Verification items for the finished model (mm, model axes). A direction names the side the tool comes from. Round coordinates to 2 decimals unless told otherwise and drop trailing zeros. Write each loop counter-clockwise with the first axis right and the second up, starting at its lowest first coordinate (ties: lowest second). Pieces come first, ordered by that corner, then holes. Notation, with made-up numbers: (-18, -32) -> (9, -32) arc R30 ccw to (9, -4) -> close; hole circle Ø9 at (9.5, 20). An arc over 180 degrees is marked (long way). Answer as a JSON object with one key per item and string values. Group by question number.
(1) Sectioned sample at B-B on y = 21.5. Record the cut outline in (x, z).
(2) Sectioned sample at A-A on z = 14. Record the cut outline in (x, y).
(3) Draft check along X on faces 5 (the face through (35, 15, 14)), 6 (the face through (6, 30, 14)), 7 (the face through (6.11, 16.01, 4.93)). Enter one of: released by +X, released by -X, zero draft, split by the parting line, or undercut.
(4) Scan lines: L1, parallel to Y at x = 5.5, z = 23.25; L2, parallel to Z at x = 17.5, y = 23; L3, parallel to X at y = 18.75, z = 14. Record each from-to range of solid material in increasing order. Write a range as from..to.
(5) Sectioned sample at C-C on x = 22. Record the cut outline in (y, z).
(6) Gauge pin test, flat ends, axial feed: pin 1 Ø3 at (x, y) = (5.5, 24) entering from +Z; pin 2 Ø6.5 at (x, z) = (16, 10.5) entering from +Y; pin 3 Ø1.5 at (x, z) = (25, 13.5) entering from +Y. Record the tip position at first contact, or that the pin passes through.
(7) Sectioned sample at D-D on y = 12. Record the cut outline in (x, z).
(8) Set-up check for faces 1 (the face through (31.408, 6.601, 24.549)), 2 (the face through (23, 8, 17)), 3 (the face through (16, 21, 6)), 4 (the face through (5, 15, 10)): record each of +Z, -Z, +X, -X, +Y, -Y from which the full face is reachable in a straight line by a thin tool's end or side.
```python
from build123d import *

# Parameters (mm, degrees)
SKETCH1_W           = 35
SKETCH1_H           = 30
BOSS_EXTRUDE1_DEPTH = 28
SKETCH2_R           = 2
CUT_EXTRUDE1_DEPTH  = 7
SKETCH4_R           = 7
CUT_EXTRUDE2_DEPTH  = 8
SKETCH5_R           = 6
CUT_EXTRUDE3_DEPTH  = 50
SKETCH6_R           = 11
CUT_EXTRUDE4_DEPTH  = 4
SKETCH7_R           = 1.5
CUT_EXTRUDE5_DEPTH  = 10
SKETCH8_R           = 1.5
CUT_EXTRUDE6_DEPTH  = 10


with BuildPart() as part:
    # Sketch1 → Boss-Extrude1 (new body)
    with BuildSketch(Plane.XY):
        with Locations((17.5, 15)):
            Rectangle(SKETCH1_W, SKETCH1_H)
    extrude(amount=BOSS_EXTRUDE1_DEPTH)

    # Sketch2 → Cut-Extrude1 (cut)
    with BuildSketch(Plane.XY.offset(28)):
        with Locations((5.5, 24)):
            Circle(SKETCH2_R)
        with Locations((5.5, 6)):
            Circle(SKETCH2_R)
        with Locations((29.5, 6)):
            Circle(SKETCH2_R)
        with Locations((29.5, 24)):
            Circle(SKETCH2_R)
    extrude(amount=-CUT_EXTRUDE1_DEPTH, mode=Mode.SUBTRACT)

    # Sketch4 → Cut-Extrude2 (cut)
    with BuildSketch(Plane.XZ):
        with Locations((17.5, 14)):
            Circle(SKETCH4_R)
    extrude(amount=-CUT_EXTRUDE2_DEPTH, mode=Mode.SUBTRACT)

    # Sketch5 → Cut-Extrude3 (cut)
    with BuildSketch(Plane(origin=(0, 8, 0), x_dir=(-1, 0, 0), z_dir=(0, -1, 0))):
        with Locations((-17.5, -14)):
            Circle(SKETCH5_R)
    extrude(amount=-CUT_EXTRUDE3_DEPTH, mode=Mode.SUBTRACT)

    # Sketch6 → Cut-Extrude4 (cut)
    with BuildSketch(Plane(origin=(0, 30, 0), x_dir=(1, 0, 0), z_dir=(0, 1, 0))):
        with Locations((17.5, -14)):
            Circle(SKETCH6_R)
    extrude(amount=-CUT_EXTRUDE4_DEPTH, mode=Mode.SUBTRACT)

    # Sketch7 → Cut-Extrude5 (cut)
    with BuildSketch(Plane(origin=(0, 26, 0), x_dir=(1, 0, 0), z_dir=(0, 1, 0))):
        with Locations((17.5, -6)):
            Circle(SKETCH7_R)
        with Locations((9.5, -14)):
            Circle(SKETCH7_R)
        with Locations((17.5, -22)):
            Circle(SKETCH7_R)
        with Locations((25.5, -14)):
            Circle(SKETCH7_R)
    extrude(amount=-CUT_EXTRUDE5_DEPTH, mode=Mode.SUBTRACT)

    # Sketch8 → Cut-Extrude6 (cut)
    with BuildSketch(Plane(origin=(0, 0, 0), x_dir=(-1, 0, 0), z_dir=(0, 0, -1))):
        with Locations((-5, 15)):
            Circle(SKETCH8_R)
    extrude(amount=-CUT_EXTRUDE6_DEPTH, mode=Mode.SUBTRACT)


solid = part.part
```
Computed values:
{
 "1": {"outline": "(0, 0) -> (35, 0) -> (35, 28) -> (0, 28) -> close; hole circle Ø3 at (9.5, 14); hole circle Ø12 at (17.5, 14); hole circle Ø3 at (17.5, 6); hole circle Ø3 at (17.5, 22); hole circle Ø3 at (25.5, 14)"},
 "2": {"outline": "(0, 0) -> (10.5, 0) -> (10.5, 8) -> (11.5, 8) -> (11.5, 26) -> (11, 26) -> (11, 16) -> (8, 16) -> (8, 26) -> (6.5, 26) -> (6.5, 30) -> (0, 30) -> close; (23.5, 8) -> (24.5, 8) -> (24.5, 0) -> (35, 0) -> (35, 30) -> (28.5, 30) -> (28.5, 26) -> (27, 26) -> (27, 16) -> (24, 16) -> (24, 26) -> (23.5, 26) -> close"},
 "3": {"face 5": "released by +X", "face 6": "zero draft", "face 7": "undercut"},
 "4": {"L1": "0..4, 8..22, 26..30", "L2": "0..4.5, 7.5..8, 20..20.5, 23.5..28", "L3": "0..8, 11..11.5, 23.5..24, 27..35"},
 "5": {"outline": "(0, 0) -> (30, 0) -> (30, 3.96) -> (26, 3.96) -> (26, 10.03) -> (8, 10.03) -> (8, 8.64) -> (0, 8.64) -> close; (0, 19.36) -> (8, 19.36) -> (8, 17.97) -> (26, 17.97) -> (26, 24.04) -> (30, 24.04) -> (30, 28) -> (0, 28) -> close"},
 "6": {"pin 1": "z = 21", "pin 2": "y = 26", "pin 3": "y = 16"},
 "7": {"outline": "(0, 0) -> (35, 0) -> (35, 28) -> (0, 28) -> close; hole circle Ø12 at (17.5, 14)"},
 "8": {"face 1": "+Z", "face 2": "-Y", "face 3": "+Y", "face 4": "-Z"}
}
